For this review, take the finished solid that the model builds, in its own axes (mm). A direction names the side the tool comes from. Round coordinates to 2 decimals unless told otherwise and drop trailing zeros. Order: outer loops, then holes, each group sorted by start corner. A loop starts at its lowest first (then second) coordinate and runs counter-clockwise, first axis right, second up. Notation, with made-up numbers: M -23.75,33.25 L -8.75,33.25 A31 ccw -8.75,70.25 Z; hole C 32,39.5 d7. An arc over 180 degrees is marked long. Answer as a JSON object with one key per item and string values.
from build123d import *

# Parameters (mm, degrees)
SKETCH2_R                 = 6
BOSS_EXTRUDE1_DEPTH       = 6.3
SKETCH3_R                 = 3
BOSS_EXTRUDE2_DEPTH       = 15.5
M3X0_5_TAPPED_HOLE1_D     = 2.5
M3X0_5_TAPPED_HOLE1_DEPTH = 3.5
M3X0_5_TAPPED_HOLE1_TIP   = 0.751075774
CUT_EXTRUDE1_START        = -12
CUT_EXTRUDE1_DEPTH        = 12


with BuildPart() as part:
    # Sketch1 → Revolve1 (revolve)
    with BuildSketch(Plane(origin=(0, 0, 0), x_dir=(0, 0, -1), z_dir=(1, 0, 0)), mode=Mode.PRIVATE) as revolve1_sk:
        Polygon((0, 0), (0, -1.5), (3, -1.5), (3, -5.5), (6, -5.5), (6, -18), (57, -18), (57, -18.5), (85, -18.5), (85, 0), align=None)
    revolve(revolve1_sk.sketch.rotate(Axis((0, 0, -33.870967742), (0, 0, 1)), 270), axis=Axis((0, 0, -33.870967742), (0, 0, 1)))

    # Sketch2 → Boss-Extrude1 (add)
    with BuildSketch(Plane(origin=(0, 0, -85), x_dir=(-1, 0, 0), z_dir=(0, 0, -1))):
        with Locations(Location((0, 7, 0), (0, 0, 180))):
            Circle(SKETCH2_R)
    extrude(amount=BOSS_EXTRUDE1_DEPTH)

    # Sketch3 → Boss-Extrude2 (add)
    with BuildSketch(Plane(origin=(0, 0, -91.3), x_dir=(-1, 0, 0), z_dir=(0, 0, -1))):
        with Locations((0, 7)):
            Circle(SKETCH3_R)
    extrude(amount=BOSS_EXTRUDE2_DEPTH)

    # M3x0.5 Tapped Hole1
    with Locations(Plane(origin=(0, 0, -85), x_dir=(-1, 0, 0), z_dir=(0, 0, -1))):
        with Locations((7.75, -13.423393759), (15.5, 0), (-15.5, 0), (7.75, 13.423393759)):
            Hole(M3X0_5_TAPPED_HOLE1_D / 2, depth=M3X0_5_TAPPED_HOLE1_DEPTH)
            with Locations((0, 0, -(M3X0_5_TAPPED_HOLE1_DEPTH + M3X0_5_TAPPED_HOLE1_TIP / 2))):  # 118° drill point
                Cone(0, M3X0_5_TAPPED_HOLE1_D / 2, M3X0_5_TAPPED_HOLE1_TIP, mode=Mode.SUBTRACT)

    # Sketch6 → Cut-Extrude1 (cut)
    with BuildSketch(Plane(origin=(0, 0, -106.8), x_dir=(-1, 0, 0), z_dir=(0, 0, -1)).offset(CUT_EXTRUDE1_START)):
        with BuildLine():
            Line((-1.658312395, 4.5), (1.658312395, 4.5))
            ThreePointArc((1.658312395, 4.5), (0, 4), (-1.658312395, 4.5))
        make_face()
    extrude(amount=CUT_EXTRUDE1_DEPTH, mode=Mode.SUBTRACT)


solid = part.part
1) Machinability: for faces 1 (the flat face through (4.02, 17.73, -57)), 2 (the flat face through (0, 0, 0)), 3 (the flat face through (0, 4.5, -101)), 4 (the cylindrical face through (0, 10, -99)), which of the approach directions +Z, -Z, +X, -X, +Y, -Y give a long, thin tool a straight path to every point of the face, cutting with its end or side? Answer none if there is none.
Geometry check:
{"face 1": "+Z", "face 2": "+Z, +X, -X, +Y, -Y", "face 3": "-Z, +X, -X, -Y", "face 4": "-Z"}
2) Add section B-B on y = -16. State the section outline as (x, z) points, and give its area (3 significant figures).
Geometry check:
{"outline": "M -9.29,-85 L 9.29,-85 L 9.29,-57 L 8.25,-57 L 8.25,-6 L -8.25,-6 L -8.25,-57 L -9.29,-57 Z", "area": "1,360 mm²"}
3) Add section D-D on x = 10. State the section outline as (y, z) points, and give its area (3 significant figures).
Geometry check:
{"outline": "M -15.56,-85 L 15.56,-85 L 15.56,-57 L 14.97,-57 L 14.97,-6 L -14.97,-6 L -14.97,-57 L -15.56,-57 Z", "area": "2,400 mm²"}
4) For L1, parallel to Y at x = -7.75, z = -83.4; L2, parallel to Z at x = -4.5, y = -11; L3, parallel to Z at x = 4.5, y = 2, list the stretches that pass through material, from the lowest coordinate up.
Geometry check:
{"L1": "y = -16.8 to -14.67, -12.17 to 12.17, 14.67 to 16.8", "L2": "z = -85 to -6", "L3": "z = -85 to -3"}
5) Mouldability with a two-part tool opening along Y and no side actions: class faces 5 (the flat face through (0, 7, -106.8)), 6 (the cylindrical face through (-16.75, 0.05, -83.23)), 7 (the cylindrical face through (-1.43, -0.45, -1.52)) as +Y half, -Y half, draft (parallel to the pull), parting line (faces both ways), or undercut.
Geometry check:
{"face 5": "draft", "face 6": "undercut", "face 7": "parting line"}
6) Add section C-C on z = -79. State the section outline as (x, y) points.
Geometry check:
{"outline": "C 0,0 d37"}
7) Insertion check: P1, Ø8, axis at x = -13.5, y = 6.5, coming from the -Z side; P2, Ø3.5, axis at x = 0, z = -101, coming from the -Y side; P3, Ø6, axis at x = 12, z = -51.5, coming from the -Y side. Each pin has a flat end and moves straight along its axis. Give the tip position at first contact, or say it passes through.
Geometry check:
{"P1": "stops at z = -85", "P2": "stops at y = 4.5", "P3": "stops at y = -15.59"}
8) Add section A-A on x = 0. State the section outline as (y, z) points.
Geometry check:
{"outline": "M -18.5,-85 L 1,-85 L 1,-91.3 L 4,-91.3 L 4,-94.8 L 4.5,-94.8 L 4.5,-106.8 L 10,-106.8 L 10,-91.3 L 13,-91.3 L 13,-85 L 18.5,-85 L 18.5,-57 L 18,-57 L 18,-6 L 5.5,-6 L 5.5,-3 L 1.5,-3 L 1.5,0 L -1.5,0 L -1.5,-3 L -5.5,-3 L -5.5,-6 L -18,-6 L -18,-57 L -18.5,-57 Z"}
